Can you work these out from the model? Positions are in its coordinate system, mm. Face numbers are marked on the shaded views. Give positions to 0.01 mm unless a question says otherwise; leave off trailing zeros. Loops run counter-clockwise (first coordinate to the right, second up) from the corner with the lowest first, then second, coordinate; pieces in that order, holes last. Notation, with made-up numbers: M 57,-19.75 L 116,-19.75 A22 cw 116,16.25 Z; hole C 58,55 d8. An arc over 180 degrees is marked long. Use CSV: the item, a comma, the result in double quotes.
from build123d import *

# Parameters (mm, degrees)
ESQUISSE1_R             = 30
BOSS_EXTRU_1_DEPTH      = 6.35
ENL_V_MAT_EXTRU_1_REACH = 44.899
ESQUISSE2_R             = 3.175
SKETCH1_R               = 1.8288
CUT_EXTRUDE1_DEPTH      = 6.35
CIRPATTERN1_COUNT       = 4


with BuildPart() as part:
    # Esquisse1 → Boss.-Extru.1 (new body)
    with BuildSketch(Plane(origin=(0, 0, 0), x_dir=(1, 0, 0), z_dir=(0, 1, 0))):
        with Locations(Location((0, 0, 0), (0, 0, 270))):
            Circle(ESQUISSE1_R)
    extrude(amount=BOSS_EXTRU_1_DEPTH)

    # Esquisse2 → Enlèv. mat.-Extru.1 (cut, up to next)
    with BuildSketch(Plane(origin=(0, 6.35, 0), x_dir=(1, 0, 0), z_dir=(0, 1, 0)), mode=Mode.PRIVATE) as enl_v_mat_extru_1_sk1:
        with Locations(Location((0, 0, 0), (0, 0, 270))):
            Circle(ESQUISSE2_R)
    enl_v_mat_extru_1_tool1 = extrude(enl_v_mat_extru_1_sk1.sketch, amount=-ENL_V_MAT_EXTRU_1_REACH, mode=Mode.PRIVATE) & part.part
    add(enl_v_mat_extru_1_tool1.solids().sort_by_distance((0, 6.35, 0))[0], mode=Mode.SUBTRACT)

    # Sketch1 → Cut-Extrude1 (cut)
    with BuildSketch(Plane(origin=(0, 6.35, 0), x_dir=(1, 0, 0), z_dir=(0, 1, 0))):
        with Locations(Location((-6.914797213, -6.914797213, 0), (0, 0, 270))):
            Circle(SKETCH1_R)
    cut_extrude1 = extrude(amount=-CUT_EXTRUDE1_DEPTH, mode=Mode.SUBTRACT)

    # CirPattern1: Cut-Extrude1 ×4 about axis
    cirpattern1_axis = Axis((0, 0, 0), (0, 1, 0))
    for i in range(1, CIRPATTERN1_COUNT):
        add(cut_extrude1.rotate(cirpattern1_axis, i * 360 / CIRPATTERN1_COUNT), mode=Mode.SUBTRACT)


solid = part.part
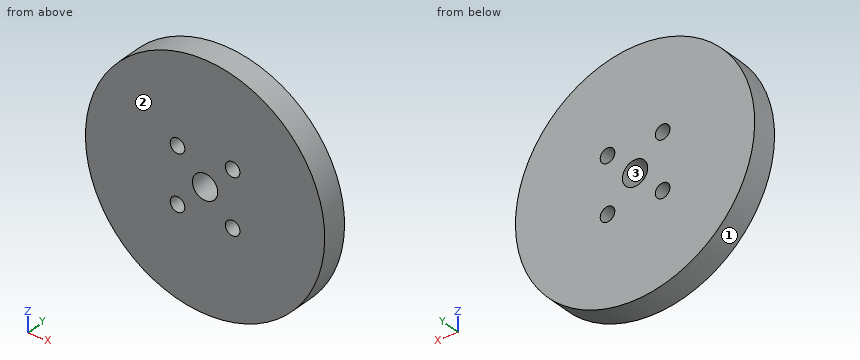
Q1. I want a section at B-B, the plane x = 0. Please give me the cut outline in (y, z) (3 decimals), then the cut area to 3 significant figures.
Model answer:
outline,"M 0,-30 L 6.35,-30 L 6.35,-3.175 L 0,-3.175 Z; M 0,3.175 L 6.35,3.175 L 6.35,30 L 0,30 Z"
area,"341 mm2"
Q2. I want a section at C-C, the plane y = 2. Please give me the cut outline in (x, z) (3 decimals).
Model answer:
outline,"C 0,0 d60; hole C -6.915,-6.915 d3.658; hole C -6.915,6.915 d3.658; hole C 0,0 d6.35; hole C 6.915,-6.915 d3.658; hole C 6.915,6.915 d3.658"
Q3. I want a section at A-A, the plane z = 0. Please give me the cut outline in (x, y) (3 decimals), then the cut area to 3 significant figures.
Model answer:
outline,"M -30,0 L -3.175,0 L -3.175,6.35 L -30,6.35 Z; M 3.175,0 L 30,0 L 30,6.35 L 3.175,6.35 Z"
area,"341 mm2"
Q4. If we mould it in two halves opening along Z, with no side actions, what happens to the marked faces 1, 2 and 3? For each: released by +Z, released by -Z, zero draft, split by the parting line, or undercut.
Model answer:
face 1,"split by the parting line"
face 2,"zero draft"
face 3,"undercut"
Q5. Please list where these lines run through material, in increasing order: L1, parallel to Z at x = -8, y = 3; L2, parallel to Z at x = 7, y = 5.25; L3, parallel to X at y = 2.75, z = -8.5. Write a range as from..to.
Model answer:
L1,"-28.91..-8.39, -5.44..5.44, 8.39..28.91"
L2,"-29.17..-8.74, -5.09..5.09, 8.74..29.17"
L3,"-28.77..-7.83, -6..6, 7.83..28.77"
Q6. I want a section at D-D, the plane z = -24. Please give me the cut outline in (x, y), then the cut area to 3 significant figures.
Model answer:
outline,"M -18,0 L 18,0 L 18,6.35 L -18,6.35 Z"
area,"229 mm2"
Q7. I'm going to push a flat-ended pin straight in: P1, Ø3, axis at x = -6.91, z = -6.91, coming from the +Y side. Where does the tip first touch, or does it pass through?
Model answer:
P1,"through"
